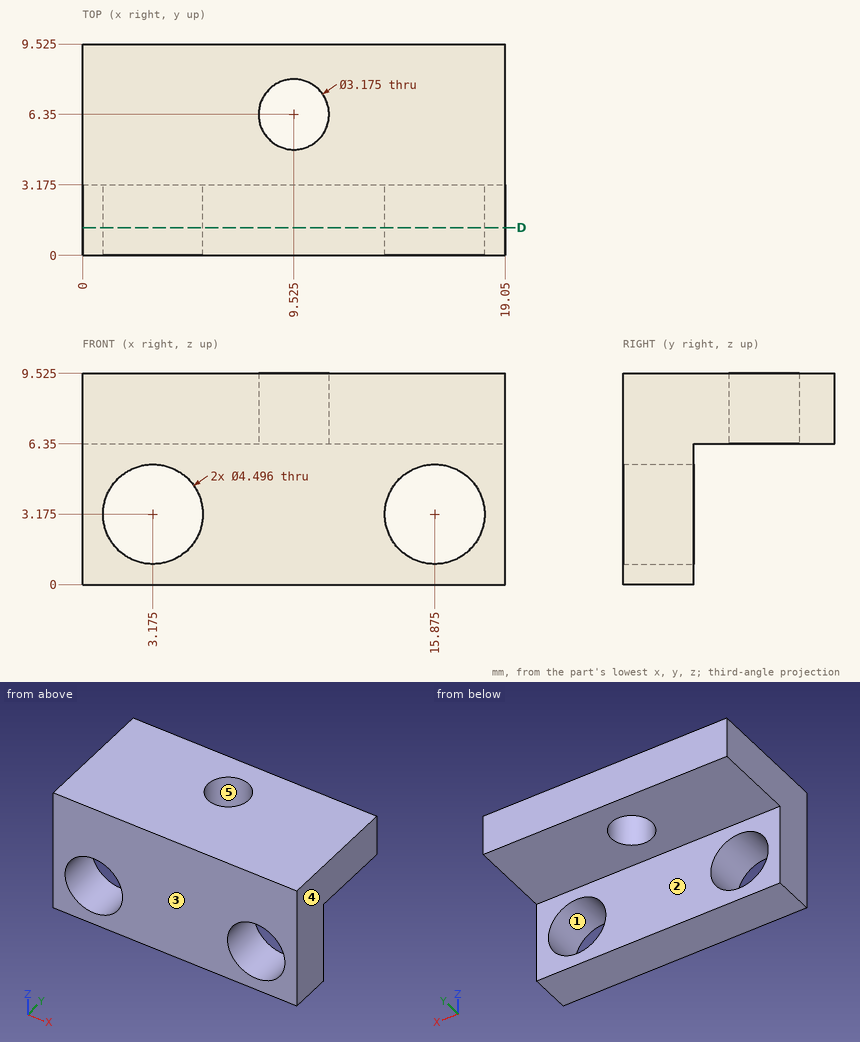
Geometry check sheet. Reference: drawing and pictorial views, mm from the part's lowest x, y, z. A direction names the side the tool comes from. Round coordinates to 2 decimals unless told otherwise and drop trailing zeros. One line per question, with ' | ' between items. Start each with the question number.
1. Sectioned sample at D-D, the plane y = 1.25. Count the separate pieces of the cut face and the enclosed holes in it, then the cut area to 3 significant figures.
2. Release check for a two-part mould opening along X. For the marked faces 3, 4 and 5 record: +X half, -X half, draft (parallel to the pull), parting line (faces both ways), or undercut.
3. Depth check by flat-ended pin: pin 1 (2.5 mm diameter, centred on x = 3.175, z = 3.175, fed in from +Y); pin 2 (4 mm diameter, centred on x = 3.5, z = 3.5, fed in from +Y) (3 decimals); pin 3 (5 mm diameter, centred on x = 6.5, y = 8, fed in from -Z). Enter the tip coordinate at first touch or a pass-through.
4. Set-up check for the marked faces 1 and 2: record each of +Z, -Z, +X, -X, +Y, -Y from which the full face is reachable in a straight line by a thin tool's end or side.
5. Scan lines: line 1 along X through (y, z) = (2.5, 3); line 2 along Y through (x, z) = (5.5, 5.75) (3 decimals); line 3 along Z through (x, y) = (2, 8.75) (3 decimals). Record each from-to range of solid material in increasing order. Write a range as from..to.
Taken from the geometry:
1) separate pieces: 1 | enclosed holes: 2 | area: 150 mm^2
2) face 3: draft | face 4: +X half | face 5: undercut
3) pin 1: passes through | pin 2: stops at y = 3.175 | pin 3: stops at z = 6.35
4) face 1: +Y, -Y | face 2: -Z, +X, -X, +Y
5) line 1: x = 0..0.93, 5.42..13.63, 18.12..19.05 | line 2: y = 0..3.175 | line 3: z = 6.35..9.525
